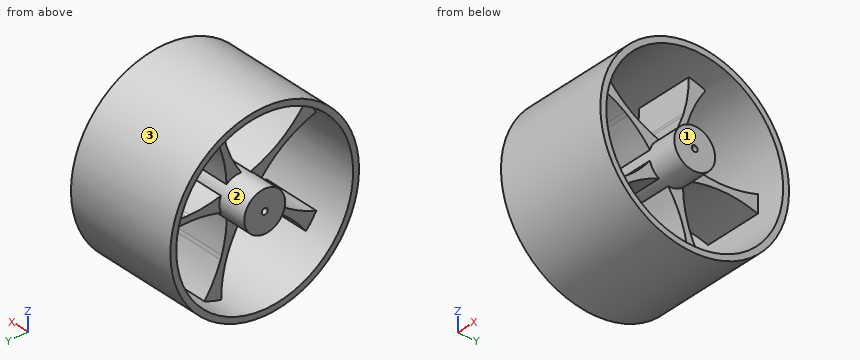
```python
from build123d import *

# Parameters (mm, degrees)
SKETCH1_R           = 80
SKETCH1_R_2         = 75
SKETCH1_R_3         = 15
SKETCH1_R_4         = 17.320508076
BOSS_EXTRUDE1_DEPTH = 100
BOSS_EXTRUDE2_START = -25
BOSS_EXTRUDE2_DEPTH = 50
SKETCH6_R           = 2.5
CUT_EXTRUDE1_DEPTH  = 100
CIRPATTERN1_COUNT   = 5


with BuildPart() as part:
    # Sketch1 → Boss-Extrude1 (new body)
    with BuildSketch(Plane(origin=(0, 0, 0), x_dir=(0, 0, -1), z_dir=(1, 0, 0))):
        Circle(SKETCH1_R)
        Circle(SKETCH1_R_2, mode=Mode.SUBTRACT)
        Circle(SKETCH1_R_3)
        Polygon((-17.320508076, 0), (-8.660254038, -15), (8.660254038, -15), (17.320508076, 0), (8.660254038, 15), (-8.660254038, 15), align=None)
        Circle(SKETCH1_R_4)
    extrude(amount=BOSS_EXTRUDE1_DEPTH)

    # Sketch7 → Boss-Extrude2 (add)
    with BuildSketch(Plane.ZY.offset(BOSS_EXTRUDE2_START)):
        with BuildLine():
            add(Edge.make_bspline(
                [(6.440327224, 16.078625105), (2.594720076, 29.237330687), (2.383712029, 42.366824241)],
                knots=[0.048824519, 0.048824519, 0.048824519, 0.47524405, 0.47524405, 0.47524405], degree=2))
            add(Edge.make_bspline(
                [(2.383712029, 42.366824241), (2.359211722, 43.891299831), (2.383712029, 45.415381593)],
                knots=[0.47524405, 0.47524405, 0.47524405, 0.52475595, 0.52475595, 0.52475595], degree=2))
            add(Edge.make_bspline(
                [(2.383712029, 45.415381593), (2.618880242, 60.044406046), (7.368611427, 74.637146017)],
                knots=[0.52475595, 0.52475595, 0.52475595, 1, 1, 1], degree=2))
            ThreePointArc((7.368611427, 74.637146017), (-0.131481233, 74.999884751), (-7.630255972, 74.610851716))
            add(Edge.make_bspline(
                [(-6.683078321, 15.979251051), (1.926800998, 45.372338084), (-7.630255972, 74.610851716)],
                knots=[0.049553835, 0.049553835, 0.049553835, 1, 1, 1], degree=2))
            ThreePointArc((-6.683078321, 15.979251051), (-4.684644195, 16.674954536), (-2.616287971, 17.121770856))
            ThreePointArc((-2.616287971, 17.121770856), (-0.117518624, 17.320109393), (2.383712029, 17.155696342))
            ThreePointArc((2.383712029, 17.155696342), (4.444765212, 16.740491695), (6.440327224, 16.078625105))
        make_face()
    boss_extrude2 = extrude(amount=-BOSS_EXTRUDE2_DEPTH)

    # Sketch6 → Cut-Extrude1 (cut)
    with BuildSketch(Plane.ZY):
        Circle(SKETCH6_R)
    extrude(amount=-CUT_EXTRUDE1_DEPTH, mode=Mode.SUBTRACT)

    # CirPattern1: Boss-Extrude2 ×5 about axis
    cirpattern1_axis = Axis((100, 0, 0), (-1, 0, 0))
    for i in range(1, CIRPATTERN1_COUNT):
        add(boss_extrude2.rotate(cirpattern1_axis, i * 360 / CIRPATTERN1_COUNT))


solid = part.part
```
Verification items for the finished model (mm, model axes). Face numbers are marked on the shaded views. Round coordinates to 2 decimals unless told otherwise and drop trailing zeros. Order: outer loops, then holes, each group sorted by start corner. A loop starts at its lowest first (then second) coordinate and runs counter-clockwise, first axis right, second up.
1) Draft check along Y on the marked faces 1, 2 and 3. Enter one of: +Y half, -Y half, draft (parallel to the pull), parting line (faces both ways), or undercut.
Geometry says:
face 1: draft
face 2: undercut
face 3: parting line
2) Depth check by flat-ended pin: pin 1 (10 mm diameter, centred on y = -7.5, z = -24, fed in from -X); pin 2 (14 mm diameter, centred on y = -26, z = -26, fed in from +X); pin 3 (5 mm diameter, centred on x = 36, y = 45.5, fed in from -Z); pin 4 (6 mm diameter, centred on x = 12, z = -47.5, fed in from +Y). Enter the tip coordinate at first touch or a pass-through.
Geometry says:
pin 1: passes through
pin 2: stops at x = 75
pin 3: stops at z = -67.46
pin 4: stops at y = 66.48
3) Cross-section at A-A, the plane z = 0. Record the cut outline in (x, y), plus the area to 3 significant figures.
Geometry says:
outline: (0, -80) - (100, -80) - (100, -75) - (0, -75) - close; (0, -17.32) - (100, -17.32) - (100, -2.5) - (0, -2.5) - close; (0, 2.5) - (100, 2.5) - (100, 17.32) - (75, 17.32) - (75, 75) - (100, 75) - (100, 80) - (0, 80) - (0, 75) - (25, 75) - (25, 17.32) - (0, 17.32) - close
area: 6,850 mm2
4) Cross-section at C-C, the plane x = 19.5. Record the cut outline in (y, z), plus the area to 3 significant figures.
Geometry says:
outline: circle Ø160 at (0, 0); circle Ø34.64 at (0, 0); hole circle Ø150 at (0, 0); hole circle Ø5 at (0, 0)
area: 3,360 mm2
5) Cross-section at B-B, the plane y = -70. Record the cut outline in (x, z).
Geometry says:
outline: (0, -38.73) - (100, -38.73) - (100, -26.93) - (0, -26.93) - close; (0, 26.93) - (100, 26.93) - (100, 38.73) - (0, 38.73) - close
6) Cross-section at D-D, the plane y = 47.5. Give the number of separate pieces and of enclosed holes in the cut face, plus the area to 3 significant figures.
Geometry says:
separate pieces: 3
enclosed holes: 0
area: 1,520 mm2
7) Material ranges on line 1 (Y direction, x = 46.5, z = 0); line 2 (Z direction, x = 71.5, y = -14); line 3 (Z direction, x = 65.5, y = 45), recorded low to high.
Geometry says:
line 1: y = -80 to -75, -17.32 to -2.5, 2.5 to 80
line 2: z = -78.77 to -73.68, -16.5 to 16.73, 73.68 to 78.77
line 3: z = -66.14 to -60, -2.61 to 2.38, 60 to 66.14
